Work out the finished part from the listing and answer in its coordinate system (mm). Round coordinates to 2 decimals unless told otherwise and drop trailing zeros. Order: outer loops, then holes, each group sorted by start corner. A loop starts at its lowest first (then second) coordinate and runs counter-clockwise, first axis right, second up. Notation, with made-up numbers: M 3.5,63.25 L 32.5,63.25 A15 ccw 32.5,81.25 Z; hole C -15.5,-11 d11. An arc over 180 degrees is marked long. Return JSON: item names as keys, results as strings.
from build123d import *

# Parameters (mm, degrees)
SKETCH_1_W          = 50
SKETCH_1_H          = 85
EXTRUDE_1_DEPTH     = 3
FILLET_2_R          = 10
SKETCH_4_R          = 1.5
CUT_EXTRUDE_1_DEPTH = 3
CHAMFER_1_SIZE      = 0.5
CUT_EXTRUDE_3_DEPTH = 3
SKETCH_7_R          = 22.5
CUT_EXTRUDE_4_DEPTH = 3
FILLET_4_R          = 4


with BuildPart() as part:
    # 草图1 → 凸台-拉伸1 (new body)
    with BuildSketch(Plane(origin=(0, 0, 0), x_dir=(0, 0, -1), z_dir=(1, 0, 0))):
        with Locations((0, 7.5)):
            Rectangle(SKETCH_1_W, SKETCH_1_H)
    extrude(amount=EXTRUDE_1_DEPTH)

    # 圆角2
    fillet_2_edges = [part.edges().sort_by_distance(p)[0] for p in [
        (1.5, -35, -25),
        (1.5, -35, 25),
    ]]
    fillet(fillet_2_edges, radius=FILLET_2_R)

    # 草图4 → 切除-拉伸1 (cut)
    with BuildSketch(Plane(origin=(3, 0, 0), x_dir=(0, 0, -1), z_dir=(1, 0, 0))):
        with Locations((20, 45)):
            Circle(SKETCH_4_R)
        with Locations((-20, 45)):
            Circle(SKETCH_4_R)
        with Locations((-18, -28)):
            Circle(SKETCH_4_R)
    extrude(amount=-CUT_EXTRUDE_1_DEPTH, mode=Mode.SUBTRACT)

    # 倒角1
    chamfer_1_edges = [part.edges().sort_by_distance(p)[0] for p in [
        (3, 12.5, -25),
        (3, 50, 0),
        (3, -35, 0),
        (3, -32.071067812, 22.071067812),
        (3, -32.071067812, -22.071067812),
        (3, 12.5, 25),
    ]]
    chamfer(chamfer_1_edges, length=CHAMFER_1_SIZE)

    # 草图6 → 切除-拉伸3 (cut)
    with BuildSketch(Plane(origin=(3, 0, 0), x_dir=(0, 0, -1), z_dir=(1, 0, 0))):
        with BuildLine():
            Line((-12.5, 50), (12.5, 50))
            Line((12.5, 50), (18.896399481, 31.551800259))
            ThreePointArc((18.896399481, 31.551800259), (0, 5), (-18.896399481, 31.551800259))
            Line((-18.896399481, 31.551800259), (-12.5, 50))
        make_face()
    extrude(amount=-CUT_EXTRUDE_3_DEPTH, mode=Mode.SUBTRACT)

    # 草图7 → 切除-拉伸4 (cut)
    with BuildSketch(Plane(origin=(3, 0, 0), x_dir=(0, 0, -1), z_dir=(1, 0, 0))):
        with Locations((0, -10)):
            Circle(SKETCH_7_R)
    extrude(amount=-CUT_EXTRUDE_4_DEPTH, mode=Mode.SUBTRACT)

    # 圆角4
    fillet_4_edges = [part.edges().sort_by_distance(p)[0] for p in [
        (1.5, 9.017857143, 12.02377269),
        (1.5, 9.017857143, -12.02377269),
    ]]
    fillet(fillet_4_edges, radius=FILLET_4_R)


solid = part.part
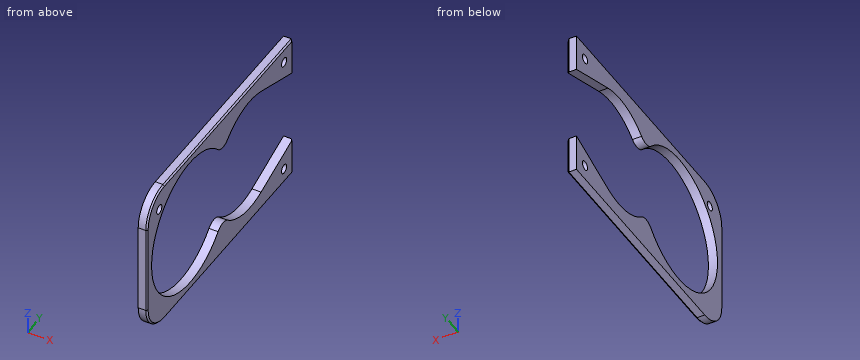
Item 1: Find section C-C (z = 0). Determine the outline of the cut face in (x, y), plus the area to 4 significant figures.
Output:
{"outline": "M 0,-35 L 2.5,-35 L 3,-34.5 L 3,-32.5 L 0,-32.5 Z", "area": "7.375 mm^2"}
Item 2: Consider line 1 along Z through (x, y) = (2.2, -10); line 2 along Y through (x, z) = (1.45, 0); line 3 along Z through (x, y) = (0.7, 32). Determine where each line is inside the solid, lowest interval first. Write a range as [from, to].
Output:
{"line 1": "z = [-25, -22.5], [22.5, 25]", "line 2": "y = [-35, -32.5]", "line 3": "z = [-25, -18.74], [18.74, 25]"}
Item 3: Find section B-B (y = 45). Determine the outline of the cut face in (x, z), plus the area to 3 significant figures.
Output:
{"outline": "M 0,-25 L 2.5,-25 L 3,-24.5 L 3,-21.5 L 0,-21.5 Z; M 0,-18.5 L 3,-18.5 L 3,-14.23 L 0,-14.23 Z; M 0,14.23 L 3,14.23 L 3,18.5 L 0,18.5 Z; M 0,21.5 L 3,21.5 L 3,24.5 L 2.5,25 L 0,25 Z", "area": "46.3 mm^2"}
Item 4: Find section D-D (x = 1.5). State how many separate pieces and enclosed holes the cut face has, plus the area to 3 significant figures.
Output:
{"separate pieces": "1", "enclosed holes": "3", "area": "1,240 mm^2"}
Item 5: Find section A-A (y = -10). Determine the outline of the cut face in (x, z), plus the area to 4 significant figures.
Output:
{"outline": "M 0,-25 L 2.5,-25 L 3,-24.5 L 3,-22.5 L 0,-22.5 Z; M 0,22.5 L 3,22.5 L 3,24.5 L 2.5,25 L 0,25 Z", "area": "14.75 mm^2"}
Item 6: This flat-tipped pin is pushed along its axis until it touches: pin 1 (2.5 mm diameter, centred on y = 45, z = -20, fed in from +X). Where does it stop, or does it pass through?
Output:
{"pin 1": "passes through"}
